The drawing under review shows one solid part. Ordinate dimensions are in mm from its lowest x, y, z. A direction names the side the tool comes from. Give positions to 0.01 mm unless a question says otherwise; leave off trailing zeros. Write each loop counter-clockwise with the first axis right and the second up, starting at its lowest first coordinate (ties: lowest second). Pieces come first, ordered by that corner, then holes. Notation, with made-up numbers: (7.25, 23.25) - (27.25, 23.25) arc R19 ccw to (27.25, 27.25) - close; hole circle Ø2 at (-6, 1). An arc over 180 degrees is marked (long way). Write item = value, one per line.
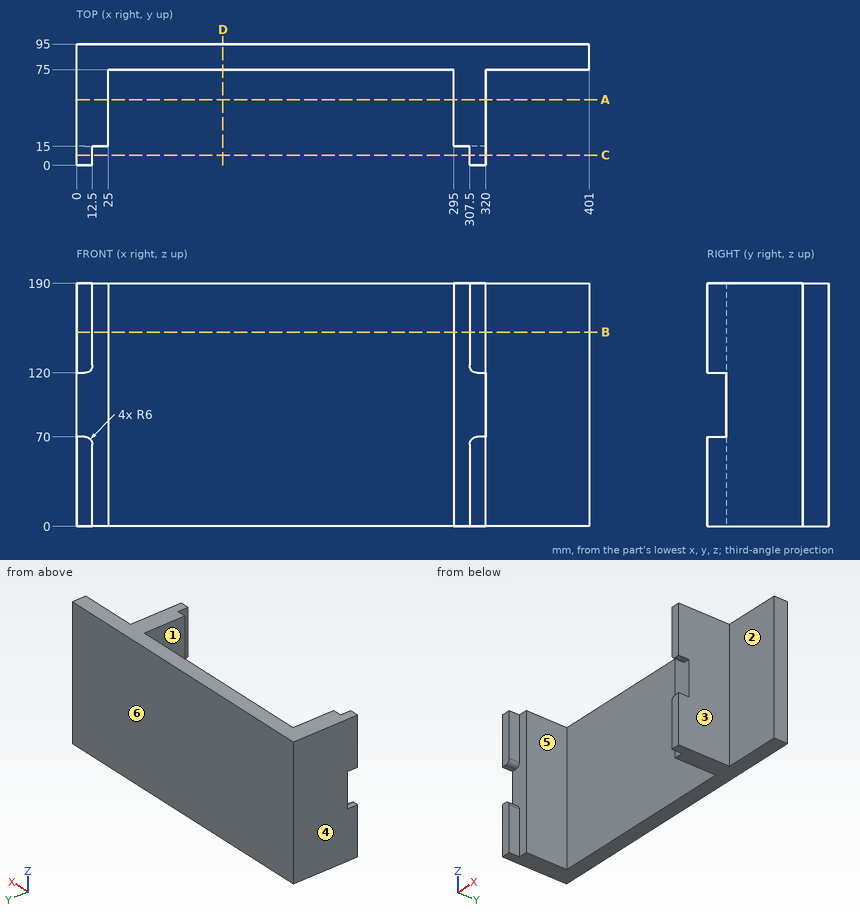
1. Draft analysis for pull direction X (two halves, no side actions). For the marked faces 1, 2, 3 and 4, state which applies: +X half, -X half, draft (parallel to the pull), parting line (faces both ways), or undercut.
Findings below:
face_1 = undercut
face_2 = draft
face_3 = +X half
face_4 = -X half
2. Insertion check: P1, Ø4, axis at y = 31, z = 77.5, coming from the +X side; P2, Ø10, axis at x = 174, y = 68, coming from the +Z side; P3, Ø7.5, axis at x = 18.5, z = 110.5, coming from the -Y side; P4, Ø24.5, axis at x = 354.5, z = 62, coming from the -Y side. Each pin has a flat end and moves straight along its axis. Give the tip position at first contact, or say it passes through.
Findings below:
P1 = 320
P2 = through
P3 = 15
P4 = 75
3. Take a section at C-C on y = 8. Give the boundary of the cut face in (x, z), and give its area (3 significant figures).
Findings below:
outline = (0, 0) - (12.5, 0) - (12.5, 64) arc R6 ccw to (6.5, 70) - (0, 70) - close; (0, 120) - (6.5, 120) arc R6 ccw to (12.5, 126) - (12.5, 190) - (0, 190) - close; (307.5, 0) - (320, 0) - (320, 70) - (313.5, 70) arc R6 ccw to (307.5, 64) - close; (307.5, 126) arc R6 ccw to (313.5, 120) - (320, 120) - (320, 190) - (307.5, 190) - close
area = 3,470 mm²
4. Take a section at A-A on y = 51.5. Give the boundary of the cut face in (x, z), and give its area (3 significant figures).
Findings below:
outline = (0, 0) - (25, 0) - (25, 190) - (0, 190) - close; (295, 0) - (320, 0) - (320, 190) - (295, 190) - close
area = 9,500 mm²
5. Take a section at D-D on x = 114.5. Give the boundary of the cut face in (y, z), and give its area (3 significant figures).
Findings below:
outline = (75, 0) - (95, 0) - (95, 190) - (75, 190) - close
area = 3,800 mm²
6. For line 1 (X direction, y = 30, z = 80); line 2 (Y direction, x = 288, z = 36), list the stretches that pass through material, from the lowest coordinate up. Write a range as from..to.
Findings below:
line_1 = 0..25, 295..320
line_2 = 75..95
7. Machinability: for the marked faces 5 and 6, which of the approach directions +Z, -Z, +X, -X, +Y, -Y give a long, thin tool a straight path to every point of the face, cutting with its end or side? Answer none if there is none.
Findings below:
face_5 = +Z, -Z, -Y
face_6 = +Z, -Z, +X, -X, +Y
8. Take a section at B-B on z = 152. Give the boundary of the cut face in (x, y).
Findings below:
outline = (0, 0) - (12.5, 0) - (12.5, 15) - (25, 15) - (25, 75) - (295, 75) - (295, 15) - (307.5, 15) - (307.5, 0) - (320, 0) - (320, 75) - (401, 75) - (401, 95) - (0, 95) - close
